from build123d import *

# Parameters (mm, degrees)
SKIZZE1_W                       = 10
SKIZZE1_H                       = 5
AUFSATZ_LINEAR_AUSTRAGEN1_DEPTH = 200
SKIZZE2_R                       = 0.6
SCHNITT_LINEAR_AUSTRAGEN1_DEPTH = 201


with BuildPart() as part:
    # Skizze1 → Aufsatz-Linear austragen1 (new body)
    with BuildSketch(Plane.XY):
        Rectangle(SKIZZE1_W, SKIZZE1_H)
    extrude(amount=AUFSATZ_LINEAR_AUSTRAGEN1_DEPTH)

    # Skizze2 → Schnitt-Linear austragen1 (cut, through all)
    with BuildSketch(Plane.XY):
        with Locations((0, -1.25)):
            Circle(SKIZZE2_R)
    extrude(amount=SCHNITT_LINEAR_AUSTRAGEN1_DEPTH, mode=Mode.SUBTRACT)


solid = part.part
Geometry: final body of the model. Coordinates: model frame, mm. Coordinates: 2 decimals unless noted, no trailing zeros. Loops run counter-clockwise (first coordinate to the right, second up) from the corner with the lowest first, then second, coordinate; pieces in that order, holes last. Notation, with made-up numbers: (60, -19) - (98, -19) arc R5 cw to (98, -10) - close; hole circle Ø5 at (-33.75, 80). An arc over 180 degrees is marked (long way). One line per question, with ' | ' between items. Start each with the question number.
(1) Draft query along Y for faces 1 (the flat face through (0, 0, 200)), 2 (the flat face through (0, -2.5, 99)), 3 (the flat face through (0, 2.5, 99)). Return one class per face: +Y half, -Y half, draft (parallel to the pull), parting line (faces both ways), or undercut.
(2) First-contact query: pin 1 (1.6 mm diameter, centred on x = 0, y = -1.25, fed in from +Z). Flat tip, straight axial feed; report the tip coordinate or a pass-through.
(3) Cut plane A-A on z = 63. Output: boundary loops of the cut face in (x, y).
(4) Ray query, L1, parallel to Y at x = 0, z = 97; L2, parallel to X at y = -1.25, z = 80.5; L3, parallel to X at y = -1.5, z = 161. Return the intervals inside material, ascending. Write a range as from..to.
Here are the results:
1) face 1: draft | face 2: -Y half | face 3: +Y half
2) pin 1: z = 200
3) outline: (-5, -2.5) - (5, -2.5) - (5, 2.5) - (-5, 2.5) - close; hole circle Ø1.2 at (0, -1.25)
4) L1: -2.5..-1.85, -0.65..2.5 | L2: -5..-0.6, 0.6..5 | L3: -5..-0.55, 0.55..5
